from build123d import *

# Parameters (mm, degrees)
SKETCH_1_R          = 8.5
EXTRUDE_1_DEPTH     = 15
SKETCH_2_R          = 3.5
CUT_EXTRUDE_1_DEPTH = 10
FILLET_1_R          = 3


with BuildPart() as part:
    # Эскиз1 → Бобышка-Вытянуть1 (new body)
    with BuildSketch(Plane(origin=(0, 0, 0), x_dir=(1, 0, 0), z_dir=(0, 1, 0))):
        Circle(SKETCH_1_R)
    extrude(amount=EXTRUDE_1_DEPTH)

    # Эскиз2 → Вырез-Вытянуть1 (cut)
    with BuildSketch(Plane.XZ):
        Circle(SKETCH_2_R)
    extrude(amount=-CUT_EXTRUDE_1_DEPTH, mode=Mode.SUBTRACT)

    # Скругление1
    fillet_1_edges = [part.edges().sort_by_distance(p)[0] for p in [
        (-8.5, 0, 0),
        (-8.5, 15, 0),
    ]]
    fillet(fillet_1_edges, radius=FILLET_1_R)


solid = part.part
Source: CAD feature listing. Evaluate the final solid. Frame: model axes, mm. A direction names the side the tool comes from. Give positions to 0.01 mm unless a question says otherwise; leave off trailing zeros. Write each loop counter-clockwise with the first axis right and the second up, starting at its lowest first coordinate (ties: lowest second). Pieces come first, ordered by that corner, then holes. Notation, with made-up numbers: M -17.5,-7 L 5.5,-7 A8 cw 5.5,-3 Z; hole C 80,-10.75 d2. An arc over 180 degrees is marked long. Return JSON: item names as keys, results as strings. Group by question number.
1) Cut plane B-B, the plane x = 0. Output: boundary loops of the cut face in (y, z), then the cut area to 3 significant figures.
2) First-contact query: pin 1 Ø2 at (x, z) = (-1, 1) entering from -Y; pin 2 Ø4 at (y, z) = (9.5, -3) entering from +X; pin 3 Ø1 at (y, z) = (4, -2) entering from -X; pin 4 Ø3 at (x, z) = (1.5, -6.5) entering from +Y. Flat tips, straight axial feed; report the tip coordinate or a pass-through.
3) Cut plane C-C, the plane y = 6.5. Output: boundary loops of the cut face in (x, z).
4) Set-up query: faces 1 (the face through (3.233, 4.93, -1.341)), 2 (the face through (0, 15, 0)). Return all of +Z, -Z, +X, -X, +Y, -Y with unobstructed straight access to the full face (end or side cutting, diameter ignored); none if empty.
5) Cut plane A-A, the plane z = 0. Output: boundary loops of the cut face in (x, y).
6) Cut plane D-D, the plane y = 11. Output: boundary loops of the cut face in (x, z), then the cut area to 3 significant figures.
7) Ray query, L1, parallel to Z at x = 0, y = 6.75; L2, parallel to X at y = 4.75, z = 0.25; L3, parallel to Y at x = 1.75, z = -2.5. Return the intervals inside material, ascending.
8) Draft query along X for faces 3 (the face through (4, 0, 0)), 4 (the face through (0, 10, 0)), 5 (the face through (4.57, 7.437, -7.167)). Return one class per face: released by +X, released by -X, zero draft, split by the parting line, or undercut.
Data:
{
 "1": {"outline": "M 0,-5.5 A3 ccw 3,-8.5 L 12,-8.5 A3 ccw 15,-5.5 L 15,5.5 A3 ccw 12,8.5 L 3,8.5 A3 ccw 0,5.5 L 0,3.5 L 10,3.5 L 10,-3.5 L 0,-3.5 Z", "area": "177 mm²"},
 "2": {"pin 1": "stops at y = 10", "pin 2": "stops at x = 8.44", "pin 3": "stops at x = -8.37", "pin 4": "stops at y = 15"},
 "3": {"outline": "C 0,0 d17; hole C 0,0 d7"},
 "4": {"face 1": "-Y", "face 2": "+Z, -Z, +X, -X, +Y"},
 "5": {"outline": "M -8.5,3 A3 ccw -5.5,0 L -3.5,0 L -3.5,10 L 3.5,10 L 3.5,0 L 5.5,0 A3 ccw 8.5,3 L 8.5,12 A3 ccw 5.5,15 L -5.5,15 A3 ccw -8.5,12 Z"},
 "6": {"outline": "C 0,0 d17", "area": "227 mm²"},
 "7": {"L1": "z = -8.5 to -3.5, 3.5 to 8.5", "L2": "x = -8.5 to -3.49, 3.49 to 8.5", "L3": "y = 10 to 15"},
 "8": {"face 3": "zero draft", "face 4": "undercut", "face 5": "split by the parting line"}
}
